```python
from build123d import *

# Parameters (mm, degrees)
SKETCH2_R           = 2.4892
BOSS_EXTRUDE1_DEPTH = 3.175
SKETCH4_R           = 2.4892
CUT_EXTRUDE1_DEPTH  = 919.047972743
SKETCH6_R           = 4
CUT_EXTRUDE3_DEPTH  = 919.045301638
CUT_EXTRUDE2_DEPTH  = 919.047972743
SKETCH7_R           = 3.2639
CUT_EXTRUDE4_DEPTH  = 919.047972743
CUT_EXTRUDE5_DEPTH  = 919.047972743


with BuildPart() as part:
    # Sketch2 → Boss-Extrude1 (new body)
    with BuildSketch(Plane(origin=(0, -119.026177706, 202.518411263), x_dir=(-1, 0, 0), z_dir=(-7.267823095607155e-15, 0.506696551391541, -0.8621244717602671))):
        with BuildLine():
            Line((21.054229278, 782.405033139), (177.875467972, 885.559604741))
            ThreePointArc((177.875467972, 885.559604741), (180.62401835, 892.051058523), (175.684594577, 897.080531077))
            ThreePointArc((175.684594577, 897.080531077), (167.933410831, 898.287628232), (160.099198372, 898.691420443))
            Line((160.099198372, 898.691420443), (-160.099198372, 898.691420443))
            ThreePointArc((-160.099198372, 898.691420443), (-167.933410831, 898.287628232), (-175.684594577, 897.080531077))
            ThreePointArc((-175.684594577, 897.080531077), (-180.62401835, 892.051058523), (-177.875467972, 885.559604741))
            Line((-177.875467972, 885.559604741), (-21.054229278, 782.405033139))
            ThreePointArc((-21.054229278, 782.405033139), (-18.86350312, 781.91408365), (-16.895725938, 782.994900685))
            ThreePointArc((-16.895725938, 782.994900685), (0, 790.780888599), (16.895725938, 782.994900685))
            ThreePointArc((16.895725938, 782.994900685), (18.86350312, 781.91408365), (21.054229278, 782.405033139))
        make_face()
        with Locations(Location((-127, 884.16502092, 0), (0, 0, 90))):
            Circle(SKETCH2_R, mode=Mode.SUBTRACT)
        with Locations(Location((-27.242242795, 806.191391474, 0), (0, 0, 90))):
            Circle(SKETCH2_R, mode=Mode.SUBTRACT)
        with Locations(Location((27.242242795, 806.191391474, 0), (0, 0, 90))):
            Circle(SKETCH2_R, mode=Mode.SUBTRACT)
        with Locations(Location((127, 884.16502092, 0), (0, 0, 90))):
            Circle(SKETCH2_R, mode=Mode.SUBTRACT)
    extrude(amount=BOSS_EXTRUDE1_DEPTH)

    # Sketch4 → Cut-Extrude1 (cut, through all)
    with BuildSketch(Plane(origin=(0, -117.417416155, 199.781166065), x_dir=(-1, 0, 0), z_dir=(-7.267823095607155e-15, 0.506696551391541, -0.8621244717602671))):
        with Locations(Location((-69.85, 890.753920443, 0), (0, 0, 90))):
            Circle(SKETCH4_R)
        with Locations(Location((-69.85, 832.016420443, 0), (0, 0, 90))):
            Circle(SKETCH4_R)
        with Locations(Location((69.85, 832.016420443, 0), (0, 0, 90))):
            Circle(SKETCH4_R)
        with Locations(Location((69.85, 890.753920443, 0), (0, 0, 90))):
            Circle(SKETCH4_R)
    extrude(amount=-CUT_EXTRUDE1_DEPTH, mode=Mode.SUBTRACT)

    # Sketch6 → Cut-Extrude3 (cut, through all)
    with BuildSketch(Plane(origin=(0, -119.026177706, 202.518411263), x_dir=(1, 0, 0), z_dir=(7.267823095607155e-15, -0.506696551391541, 0.8621244717602671))):
        with Locations(Location((-79.654, 873.291420443, 0), (0, 0, 270))):
            Circle(SKETCH6_R)
        with Locations(Location((-79.654, 847.891420443, 0), (0, 0, 270))):
            Circle(SKETCH6_R)
    extrude(amount=-CUT_EXTRUDE3_DEPTH, mode=Mode.SUBTRACT)

    # Sketch5 → Cut-Extrude2 (cut, through all)
    with BuildSketch(Plane(origin=(0, -117.417416155, 199.781166065), x_dir=(-1, 0, 0), z_dir=(-7.267823095607155e-15, 0.506696551391541, -0.8621244717602671))):
        with BuildLine():
            Line((99.215659501, 862.570038261), (99.215659501, 868.137802624))
            ThreePointArc((99.215659501, 868.137802624), (106.715659501, 873.353920443), (114.215659501, 868.137802624))
            Line((114.215659501, 868.137802624), (114.215659501, 862.570038261))
            ThreePointArc((114.215659501, 862.570038261), (106.715659501, 857.353920443), (99.215659501, 862.570038261))
        make_face()
    extrude(amount=-CUT_EXTRUDE2_DEPTH, mode=Mode.SUBTRACT)

    # Sketch7 → Cut-Extrude4 (cut, through all)
    with BuildSketch(Plane(origin=(0, -117.417416155, 199.781166065), x_dir=(-1, 0, 0), z_dir=(-7.267823095607155e-15, 0.506696551391541, -0.8621244717602671))):
        with Locations(Location((-76.975, 867.735170443, 0), (0, 0, 90))):
            Circle(SKETCH7_R)
        with Locations(Location((-96.025, 867.735170443, 0), (0, 0, 90))):
            Circle(SKETCH7_R)
    extrude(amount=-CUT_EXTRUDE4_DEPTH, mode=Mode.SUBTRACT)

    # Sketch8 → Cut-Extrude5 (cut, through all)
    with BuildSketch(Plane(origin=(0, -117.417416155, 199.781166065), x_dir=(-1, 0, 0), z_dir=(-7.267823095607155e-15, 0.506696551391541, -0.8621244717602671))):
        with BuildLine():
            Line((50.825, 891.603920443), (-50.825, 891.603920443))
            ThreePointArc((-50.825, 891.603920443), (-55.315128061, 889.744048503), (-57.175, 885.253920443))
            Line((-57.175, 885.253920443), (-57.175, 826.803920443))
            ThreePointArc((-57.175, 826.803920443), (-55.315128061, 822.313792382), (-50.825, 820.453920443))
            Line((-50.825, 820.453920443), (-37.5, 820.453920443))
            Line((-37.5, 820.453920443), (-37.5, 816.287420443))
            ThreePointArc((-37.5, 816.287420443), (-36.57006403, 814.042356413), (-34.325, 813.112420443))
            Line((-34.325, 813.112420443), (34.325, 813.112420443))
            ThreePointArc((34.325, 813.112420443), (36.57006403, 814.042356413), (37.5, 816.287420443))
            Line((37.5, 816.287420443), (37.5, 820.453920443))
            Line((37.5, 820.453920443), (50.825, 820.453920443))
            ThreePointArc((50.825, 820.453920443), (55.315128061, 822.313792382), (57.175, 826.803920443))
            Line((57.175, 826.803920443), (57.175, 885.253920443))
            ThreePointArc((57.175, 885.253920443), (55.315128061, 889.744048503), (50.825, 891.603920443))
        make_face()
    extrude(amount=-CUT_EXTRUDE5_DEPTH, mode=Mode.SUBTRACT)


solid = part.part
```
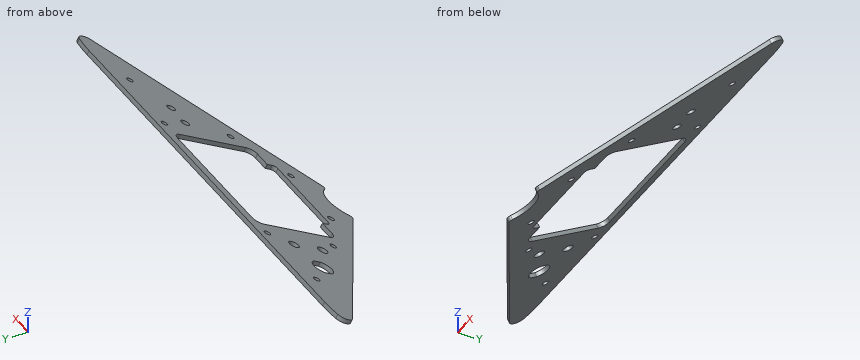
Design review of the part built by this model. Coordinates are the model's own, in mm. Round coordinates to 2 decimals unless told otherwise and drop trailing zeros. Write each loop counter-clockwise with the first axis right and the second up, starting at its lowest first coordinate (ties: lowest second). Pieces come first, ordered by that corner, then holes.
Item 1: Clearance check with flat-ended pins moving along their axes: pin 1 Ø4.5 at (y, z) = (629, 641) entering from -X; pin 2 Ø10 at (x, z) = (-6, 610) entering from -Y; pin 3 Ø5.5 at (y, z) = (587.5, 614.5) entering from -X; pin 4 Ø8 at (x, y) = (40, 594) entering from +Z. State where each tip first meets the part, or that it passes through.
Item 2: For probe 1 along Z at (x, y) = (-65, 636.5); probe 2 along X at (y, z) = (591.5, 616.5); probe 3 along Y at (x, z) = (72.5, 646), list the stretches that pass through material, from the lowest coordinate up.
Item 3: We need section B-B on x = 145. Write out the cut boundary in (y, z) (3 decimals).
Item 4: We need section A-A on x = 46.5. Write out the cut boundary in (y, z) (3 decimals), and give its area (3 significant figures).
Item 5: We need section C-C on x = -87.5. Write out the cut boundary in (y, z) (3 decimals).
Returned:
1. pin 1: stops at x = -153.19
1. pin 2: stops at y = 565.78
1. pin 3: stops at x = -79.14
1. pin 4: passes through
2. probe 1: z = 642.88 to 646.56
2. probe 2: x = -81.74 to -55.33, 55.33 to 81.74
2. probe 3: y = 635.54 to 641.81
3. outline: (625.793, 640.271) - (627.402, 637.534) - (657.366, 655.145) - (655.758, 657.882) - close
4. outline: (569.934, 607.441) - (571.543, 604.704) - (589.916, 615.502) - (588.307, 618.24) - close; (649.647, 654.291) - (651.256, 651.554) - (657.366, 655.145) - (655.758, 657.882) - close
4. area: 90.2 mm2
5. outline: (593.185, 621.107) - (594.794, 618.369) - (657.366, 655.145) - (655.758, 657.882) - close
